Job drawing, mm, ordinate dimensions from the low corner. One solid piece. A direction names the side the tool comes from. Give positions to 0.01 mm unless a question says otherwise; leave off trailing zeros. Order: outer loops, then holes, each group sorted by start corner. A loop starts at its lowest first (then second) coordinate and runs counter-clockwise, first axis right, second up. Notation, with made-up numbers: M 73.5,66.25 L 86.5,66.25 A16 ccw 86.5,85.25 Z; hole C -9.5,9.25 d11. An arc over 180 degrees is marked long. One line per question, with ' | ' between items.
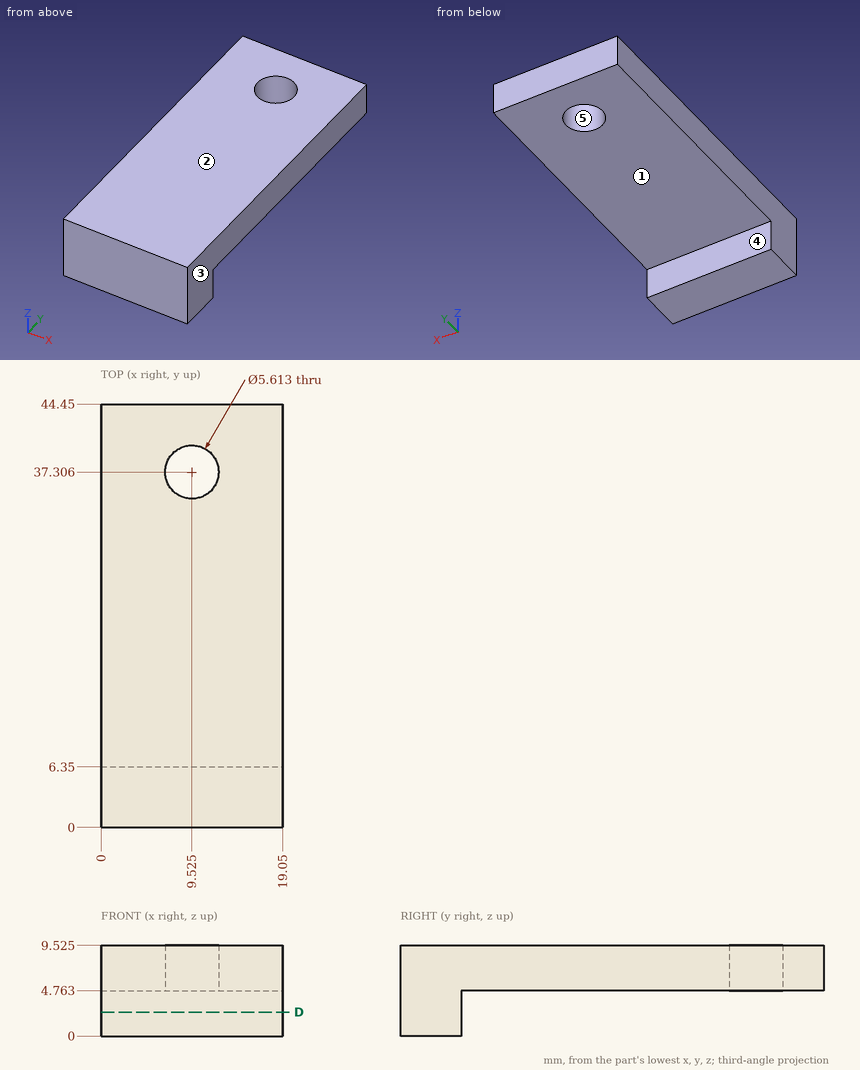
1. Tool access for the marked faces 1 and 2: list every direction of +Z, -Z, +X, -X, +Y, -Y with a clear straight run to the whole face (end or side of a thin tool).
Worked out:
face 1: -Z, +X, -X, +Y | face 2: +Z, +X, -X, +Y, -Y
2. Slice it at D-D on z = 2.5. Give the cut face in (x, y).
Worked out:
outline: M 0,0 L 19.05,0 L 19.05,6.35 L 0,6.35 Z
3. Probe L1, parallel to Z at x = 6.25, y = 36.5 (1 decimal); L2, parallel to Y at x = 5, z = 2.5. List the from-to ranges inside material, lowest first. Write a range as from..to.
Worked out:
L1: z = 4.8..9.5 | L2: y = 0..6.35
4. Mould opens along X. For the marked faces 3, 4 and 5 say: released by +X, released by -X, zero draft, split by the parting line, or undercut.
Worked out:
face 3: released by +X | face 4: zero draft | face 5: undercut
5. Drop flat-ended pins along their axis: pin 1 (5 mm diameter, centred on x = 14, z = 2, fed in from +Y); pin 2 (1 mm diameter, centred on y = 8.5, z = 2, fed in from +X). Give the stop position or say it passes through.
Worked out:
pin 1: stops at y = 6.35 | pin 2: passes through
